For this review, take the finished solid that the model builds, in its own axes (mm). Face numbers are marked on the shaded views. A direction names the side the tool comes from. Coordinates: 2 decimals unless noted, no trailing zeros. Order: outer loops, then holes, each group sorted by start corner. A loop starts at its lowest first (then second) coordinate and runs counter-clockwise, first axis right, second up. Notation, with made-up numbers: M 16.25,22 L 58.25,22 A17 ccw 58.25,52 Z; hole C 46.25,-21 d8. An arc over 180 degrees is marked long. Use one line per item in the form item = value. Start each with the question number.
```python
from build123d import *

# Parameters (mm, degrees)
BOSS_EXTRUDE1_DEPTH = 48
BOSS_EXTRUDE2_START = -3
BOSS_EXTRUDE2_DEPTH = 3
SKETCH3_W           = 75
SKETCH3_H           = 58
BOSS_EXTRUDE3_DEPTH = 3
SKETCH4_W           = 12.5
SKETCH4_H           = 12.5
CUT_EXTRUDE1_DEPTH  = 5.2


with BuildPart() as part:
    # Sketch1 → Boss-Extrude1 (new body)
    with BuildSketch(Plane.XY):
        with BuildLine():
            Line((-32.6359499, 12.129277561), (32.3640501, 12.129277561))
            Line((32.3640501, 12.129277561), (26.200760796, -3.487483918))
            ThreePointArc((26.200760796, -3.487483918), (24.961869302, -5.702906573), (23.180569313, -7.51119859))
            Line((23.180569313, -7.51119859), (22.01726547, -6.008958872))
            ThreePointArc((22.01726547, -6.008958872), (17.3640501, 7.6), (12.710834731, -6.008958872))
            Line((12.710834731, -6.008958872), (11.547530888, -7.51119859))
            ThreePointArc((11.547530888, -7.51119859), (9.766230899, -5.702906573), (8.527339405, -3.487483918))
            Line((8.527339405, -3.487483918), (7.046449616, 0.264847258))
            ThreePointArc((7.046449616, 0.264847258), (-0.1359499, 5.15176662), (-7.318349416, 0.264847258))
            Line((-7.318349416, 0.264847258), (-8.799239204, -3.487483918))
            ThreePointArc((-8.799239204, -3.487483918), (-10.038130698, -5.702906573), (-11.819430687, -7.51119859))
            Line((-11.819430687, -7.51119859), (-12.98273453, -6.008958872))
            ThreePointArc((-12.98273453, -6.008958872), (-17.6359499, 7.6), (-22.289165269, -6.008958872))
            Line((-22.289165269, -6.008958872), (-23.452469112, -7.51119859))
            ThreePointArc((-23.452469112, -7.51119859), (-25.233769101, -5.702906573), (-26.472660595, -3.487483918))
            Line((-26.472660595, -3.487483918), (-32.6359499, 12.129277561))
        make_face()
    extrude(amount=BOSS_EXTRUDE1_DEPTH)

    # Sketch2 → Boss-Extrude2 (add)
    with BuildSketch(Plane.XY.offset(48).offset(BOSS_EXTRUDE2_START)):
        with BuildLine():
            Line((22.01726547, -6.008958872), (20.058016894, -3.478870926))
            ThreePointArc((20.058016894, -3.478870926), (17.3640501, 4.4), (14.670083307, -3.478870926))
            Line((14.670083307, -3.478870926), (12.710834731, -6.008958872))
            ThreePointArc((12.710834731, -6.008958872), (17.3640501, 7.6), (22.01726547, -6.008958872))
        make_face()
        with BuildLine():
            Line((-12.98273453, -6.008958872), (-14.941983106, -3.478870926))
            ThreePointArc((-14.941983106, -3.478870926), (-17.6359499, 4.4), (-20.329916693, -3.478870926))
            Line((-20.329916693, -3.478870926), (-22.289165269, -6.008958872))
            ThreePointArc((-22.289165269, -6.008958872), (-17.6359499, 7.6), (-12.98273453, -6.008958872))
        make_face()
    extrude(amount=BOSS_EXTRUDE2_DEPTH)

    # Sketch3 → Boss-Extrude3 (add)
    with BuildSketch(Plane(origin=(0, 12.129277561, 0), x_dir=(1, 0, 0), z_dir=(0, 1, 0))):
        with Locations((-0.1359499, -24)):
            Rectangle(SKETCH3_W, SKETCH3_H)
    extrude(amount=BOSS_EXTRUDE3_DEPTH)

    # Sketch4 → Cut-Extrude1 (cut)
    with BuildSketch(Plane(origin=(0, 15.129277561, 0), x_dir=(1, 0, 0), z_dir=(0, 1, 0))):
        with Locations((21.3640501, -11)):
            Rectangle(SKETCH4_W, SKETCH4_H)
        with Locations((21.3640501, -37)):
            Rectangle(SKETCH4_W, SKETCH4_H)
        with Locations((-21.6359499, -37)):
            Rectangle(SKETCH4_W, SKETCH4_H)
        with Locations((-21.6359499, -11)):
            Rectangle(SKETCH4_W, SKETCH4_H)
    extrude(amount=-CUT_EXTRUDE1_DEPTH, mode=Mode.SUBTRACT)


solid = part.part
```
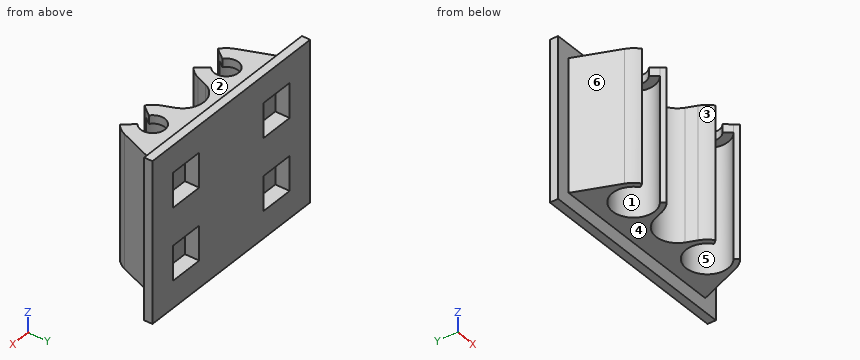
1. Consider section A-A, the plane z = 3. Write out the cut boundary in (x, y), plus the area to 3 significant figures.
2. Consider section B-B, the plane x = 30. Write out the cut boundary in (y, z), plus the area to 3 significant figures.
3. For pin 1 Ø3 at (y, z) = (2.5, 41.5) entering from +X; pin 2 Ø1.5 at (y, z) = (-0.5, 45) entering from -X; pin 3 Ø3 at (y, z) = (10.5, 23.5) entering from -X; pin 4 Ø5.5 at (x, y) = (-17.64, 0) entering from -Z, all flat-tipped, find the tip position at first contact; note any pin that passes through.
4. Tool access review of the marked faces 4, 5 and 6: name each direction out of +Z, -Z, +X, -X, +Y, -Y from which nothing blocks a thin tool from reaching the whole face with its end or side.
5. Consider section D-D, the plane x = -4. Write out the cut boundary in (y, z).
6. The part is to be moulded in two halves that separate along Y. For the marked faces 1, 2 and 3, say which applies: pulls with the +Y half, pulls with the -Y half, needs draft (parallel to the pull), parting line crosses it, or undercut.
7. Consider section C-C, the plane z = 37.5. Write out the cut boundary in (x, y).
8. To check wall thickness, follow line 1 (Z direction, x = -16.5, y = 10); line 2 (X direction, y = 0.25, z = 34); line 3 (X direction, y = 10, z = 15). State the ranges of each line that lie inside material, in increasing order.
Answers follow:
q1.outline = M -37.64,12.13 L -32.64,12.13 L -26.47,-3.49 A9.5 ccw -23.45,-7.51 L -22.29,-6.01 A7.6 cw long -12.98,-6.01 L -11.82,-7.51 A9.5 ccw -8.8,-3.49 L -7.32,0.26 A7.72 cw 7.05,0.26 L 8.53,-3.49 A9.5 ccw 11.55,-7.51 L 12.71,-6.01 A7.6 cw long 22.02,-6.01 L 23.18,-7.51 A9.5 ccw 26.2,-3.49 L 32.36,12.13 L 37.36,12.13 L 37.36,15.13 L -37.64,15.13 Z
q1.area = 782 mm²
q2.outline = M 6.14,0 L 12.13,0 L 12.13,-5 L 15.13,-5 L 15.13,53 L 12.13,53 L 12.13,48 L 6.14,48 Z
q2.area = 462 mm²
q3.pin_1 = 29.16
q3.pin_2 = -27.95
q3.pin_3 = -32.58
q3.pin_4 = through
q4.face_4 = -Z, +X, -X, -Y
q4.face_5 = -Z
q4.face_6 = +Z, -Z, -X, -Y
q5.outline = M 4.12,0 L 12.13,0 L 12.13,-5 L 15.13,-5 L 15.13,53 L 12.13,53 L 12.13,48 L 4.12,48 Z
q6.face_1 = undercut
q6.face_2 = needs draft
q6.face_3 = pulls with the -Y half
q7.outline = M -37.64,12.13 L -32.64,12.13 L -26.47,-3.49 A9.5 ccw -23.45,-7.51 L -22.29,-6.01 A7.6 cw long -12.98,-6.01 L -11.82,-7.51 A9.5 ccw -8.8,-3.49 L -7.32,0.26 A7.72 cw 7.05,0.26 L 8.53,-3.49 A9.5 ccw 11.55,-7.51 L 12.71,-6.01 A7.6 cw long 22.02,-6.01 L 23.18,-7.51 A9.5 ccw 26.2,-3.49 L 32.36,12.13 L 37.36,12.13 L 37.36,15.13 L 27.61,15.13 L 27.61,9.93 L 15.11,9.93 L 15.11,15.13 L -15.39,15.13 L -15.39,9.93 L -27.89,9.93 L -27.89,15.13 L -37.64,15.13 Z
q8.line_1 = 0 to 4.75, 17.25 to 30.75, 43.25 to 48
q8.line_2 = -27.95 to -25.23, -10.04 to -7.32, 7.05 to 9.77, 24.96 to 27.68
q8.line_3 = -31.8 to -27.89, -15.39 to 15.11, 27.61 to 31.52
